Here's how the part is built. I have some questions about the finished solid (model axes, mm). A direction names the side the tool comes from. Round coordinates to 2 decimals unless told otherwise and drop trailing zeros. Loops run counter-clockwise (first coordinate to the right, second up) from the corner with the lowest first, then second, coordinate; pieces in that order, holes last. Notation, with made-up numbers: (41, -4) -> (96, -4) arc R23 cw to (96, 21) -> close; hole circle Ø7 at (45.5, 0.25). An arc over 180 degrees is marked (long way). One line per item, written item: value. Start each with the question number.
```python
from build123d import *

# Parameters (mm, degrees)
SKETCH_1_W             = 41.5
SKETCH_1_H             = 21
EXTRUDE_346_DEPTH      = 1.6
SKETCH_2_W             = 18
SKETCH_2_H             = 11
RJ_9_DEPTH             = 12
SKETCH_3_R             = 1.25
SKETCH_3_R_2           = 1.5
CUT_EXTRUDE_1006_DEPTH = 27.968731895


with BuildPart() as part:
    # Эскиз1 → Extrude 346 (new body)
    with BuildSketch(Plane.XY):
        Rectangle(SKETCH_1_W, SKETCH_1_H)
    extrude(amount=EXTRUDE_346_DEPTH)

    # Эскиз2 → RJ-9 (add)
    with BuildSketch(Plane.XY.offset(1.6)):
        with Locations((-12.75, 0)):
            Rectangle(SKETCH_2_W, SKETCH_2_H)
    extrude(amount=RJ_9_DEPTH)

    # Эскиз3 → Cut-Extrude 1006 (cut, through all)
    with BuildSketch(Plane.XY.offset(1.6)):
        with Locations((-18, 7.5)):
            Circle(SKETCH_3_R)
        with Locations((18, 8)):
            Circle(SKETCH_3_R_2)
        with Locations(Location((18, -8, 0), (0, 0, 180))):
            Circle(SKETCH_3_R_2)
        with Locations(Location((-18, -7.5, 0), (0, 0, 180))):
            Circle(SKETCH_3_R)
    extrude(amount=-CUT_EXTRUDE_1006_DEPTH, mode=Mode.SUBTRACT)


solid = part.part
```
Q1. If I drill on line 1 along Y through (x, z) = (-18, 1); line 2 along Z through (x, y) = (16.5, 2.25); line 3 along Y through (x, z) = (-6, 11.5), over which ranges is the centre line in solid material (lowest first)?
Q2. I want a section at B-B on y = 8. Please give me the cut outline in (x, z), plus the area to 3 significant figures.
Q3. I want a section at D-D on y = -3. Please give me the cut outline in (x, z).
Q4. Will these pins go through, and if not, where does the flat tip stop? P1, Ø8, axis at x = 12.5, y = -4.5, coming from the +Z side; P2, Ø5.5, axis at y = 1.5, z = 8, coming from the +X side; P3, Ø3.5, axis at x = -13, z = 8, coming from the +Y side.
Q5. I want a section at C-C on x = 18. Please give me the cut outline in (y, z).
Q6. Which directions (+Z, -Z, +X, -X, +Y, -Y) give clear straight access to the entire face, cutting with the end or side of a thin tool? Please do faces 1 (the flat face through (-3.75, 0, 8)), 2 (the flat face through (-13, -5.5, 8)), 3 (the flat face through (-20.75, 0, 1)), 4 (the flat face through (-13, 5.5, 8)), 5 (the flat face through (0, -10.5, 1)).
Q7. I want a section at A-A on x = -18. Please give me the cut outline in (y, z), plus the area to 3 significant figures.
Q8. If we mould it in two halves opening along X, with no side actions, what happens to faces 6 (the flat face through (-13, 0, 13.6)), 7 (the cylindrical face through (16.5, 8.07, 0.81)), 8 (the flat face through (20.75, 0, 1))? For each: released by +X, released by -X, zero draft, split by the parting line, or undercut.
Answers below:
1. line 1: y = -10.5 to -8.75, -6.25 to 6.25, 8.75 to 10.5
1. line 2: z = 0 to 1.6
1. line 3: y = -5.5 to 5.5
2. outline: (-20.75, 0) -> (-19.15, 0) -> (-19.15, 1.6) -> (-20.75, 1.6) -> close; (-16.85, 0) -> (16.5, 0) -> (16.5, 1.6) -> (-16.85, 1.6) -> close; (19.5, 0) -> (20.75, 0) -> (20.75, 1.6) -> (19.5, 1.6) -> close
2. area: 57.9 mm^2
3. outline: (-21.75, 1.6) -> (-20.75, 1.6) -> (-20.75, 0) -> (20.75, 0) -> (20.75, 1.6) -> (-3.75, 1.6) -> (-3.75, 13.6) -> (-21.75, 13.6) -> close
4. P1: stops at z = 1.6
4. P2: stops at x = -3.75
4. P3: stops at y = 5.5
5. outline: (-10.5, 0) -> (-9.5, 0) -> (-9.5, 1.6) -> (-10.5, 1.6) -> close; (-6.5, 0) -> (6.5, 0) -> (6.5, 1.6) -> (-6.5, 1.6) -> close; (9.5, 0) -> (10.5, 0) -> (10.5, 1.6) -> (9.5, 1.6) -> close
6. face 1: +Z, +X, +Y, -Y
6. face 2: +Z, +X, -X, -Y
6. face 3: -Z, -X, +Y, -Y
6. face 4: +Z, +X, -X, +Y
6. face 5: +Z, -Z, +X, -X, -Y
7. outline: (-10.5, 0) -> (-8.75, 0) -> (-8.75, 1.6) -> (-10.5, 1.6) -> close; (-6.25, 0) -> (6.25, 0) -> (6.25, 1.6) -> (5.5, 1.6) -> (5.5, 13.6) -> (-5.5, 13.6) -> (-5.5, 1.6) -> (-6.25, 1.6) -> close; (8.75, 0) -> (10.5, 0) -> (10.5, 1.6) -> (8.75, 1.6) -> close
7. area: 158 mm^2
8. face 6: zero draft
8. face 7: undercut
8. face 8: released by +X
